The model under review builds one solid part; all positions refer to its coordinate system, in mm. Give positions to 0.01 mm unless a question says otherwise; leave off trailing zeros. Loops run counter-clockwise (first coordinate to the right, second up) from the corner with the lowest first, then second, coordinate; pieces in that order, holes last. Notation, with made-up numbers: (81.25, 3.25) - (96.25, 3.25) arc R17 cw to (96.25, 16.25) - close; hole circle Ø8 at (60.25, 89). An arc over 180 degrees is marked (long way). Return JSON: item names as keys, results as strings. Group by question number.
```python
from build123d import *

# Parameters (mm, degrees)
SKETCH13_R              = 4.7625
BOSS_EXTRUDE1_DEPTH     = 6.35
SKETCH14_R              = 12.7
CUT_EXTRUDE1_DEPTH      = 7.35
CUT_EXTRUDE1_DEPTH_BACK = 1
FILLET1_R               = 2.54
FILLET2_R               = 25.4


with BuildPart() as part:
    # Sketch13 → Boss-Extrude1 (new body)
    with BuildSketch(Plane(origin=(0, 0, 0), x_dir=(1, 0, 0), z_dir=(0, 1, 0))):
        with BuildLine():
            Line((12.7, 54.409872551), (25.137792916, 10.286231112))
            Line((25.137792916, 10.286231112), (13.84741683, -34.144859739))
            ThreePointArc((13.84741683, -34.144859739), (0, -44.913595269), (-13.84741683, -34.144859739))
            Line((-13.84741683, -34.144859739), (-25.137792916, 10.286231112))
            Line((-25.137792916, 10.286231112), (-12.7, 54.409872551))
            Line((-12.7, 54.409872551), (12.7, 54.409872551))
        make_face()
        with Locations((0, -30.626095269)):
            Circle(SKETCH13_R, mode=Mode.SUBTRACT)
    extrude(amount=BOSS_EXTRUDE1_DEPTH)

    # Sketch14 → Cut-Extrude1 (cut, two sides)
    with BuildSketch(Plane(origin=(0, 0, 0), x_dir=(1, 0, 0), z_dir=(0, 1, 0))) as cut_extrude1_sk:
        with Locations((0, 54.409872551)):
            Circle(SKETCH14_R)
    extrude(amount=CUT_EXTRUDE1_DEPTH, mode=Mode.SUBTRACT)
    extrude(cut_extrude1_sk.sketch, amount=-CUT_EXTRUDE1_DEPTH_BACK, mode=Mode.SUBTRACT)

    # Fillet1
    fillet1_edges = [part.edges().sort_by_distance(p)[0] for p in [
        (12.7, 3.175, -54.409872551),
        (-12.7, 3.175, -54.409872551),
    ]]
    fillet(fillet1_edges, radius=FILLET1_R)

    # Fillet2
    fillet2_edges = [part.edges().sort_by_distance(p)[0] for p in [
        (25.137792916, 3.175, -10.286231112),
        (-25.137792916, 3.175, -10.286231112),
    ]]
    fillet(fillet2_edges, radius=FILLET2_R)


solid = part.part
```
1) We need section B-B, the plane y = 5.5. Write out the cut boundary in (x, z) (1 decimal), plus the area to 3 significant figures.
2) Draft analysis for pull direction X (two halves, no side actions). For faces 1 (the face through (-12.894, 3.219, -48.222)), 2 (the face through (18.722, 3.131, 14.963)), 3 (the face through (0.26, 3.13, 44.91)), state which applies: +X half, -X half, draft (parallel to the pull), parting line (faces both ways), or undercut.
3) We need section C-C, the plane x = 18. Write out the cut boundary in (y, z), plus the area to 3 significant figures.
4) To check wall thickness, follow line 1 (Z direction, x = 0, y = 3.5); line 2 (X direction, y = 5.5, z = 30); line 3 (Z direction, x = 5, y = 5). State the ranges of each line that lie inside material, in increasing order.
5) We need section A-A, the plane x = 0. Write out the cut boundary in (y, z), plus the area to 3 significant figures.
6) For pin 1 Ø1.5 at (x, z) = (-19, -25.5) entering from -Y, flat-tipped, find the tip position at first contact; note if it passes through.
7) We need section D-D, the plane z = 16.5. Write out the cut boundary in (x, y).
Findings:
{
 "1": {"outline": "(-23.5, -3.7) arc R25.4 ccw to (-23.3, -16.8) - (-15, -46.4) arc R2.5 ccw to (-10.4, -47.2) arc R12.7 cw to (10.4, -47.2) arc R2.5 ccw to (15, -46.4) - (23.3, -16.8) arc R25.4 ccw to (23.5, -3.7) - (13.8, 34.1) arc R14.3 ccw to (-13.8, 34.1) - close; hole circle Ø9.5 at (0, 30.6)", "area": "3,270 mm^2"},
 "2": {"face 1": "undercut", "face 2": "+X half", "face 3": "parting line"},
 "3": {"outline": "(0, -35.61) - (6.35, -35.61) - (6.35, 17.8) - (0, 17.8) - close", "area": "339 mm^2"},
 "4": {"line 1": "z = -41.71 to 25.86, 35.39 to 44.91", "line 2": "x = -14.9 to -4.72, 4.72 to 14.9", "line 3": "z = -42.74 to 44.01"},
 "5": {"outline": "(0, -41.71) - (6.35, -41.71) - (6.35, 25.86) - (0, 25.86) - close; (0, 35.39) - (6.35, 35.39) - (6.35, 44.91) - (0, 44.91) - close", "area": "490 mm^2"},
 "6": {"pin 1": "stops at y = 0"},
 "7": {"outline": "(-18.33, 0) - (18.33, 0) - (18.33, 6.35) - (-18.33, 6.35) - close"}
}
